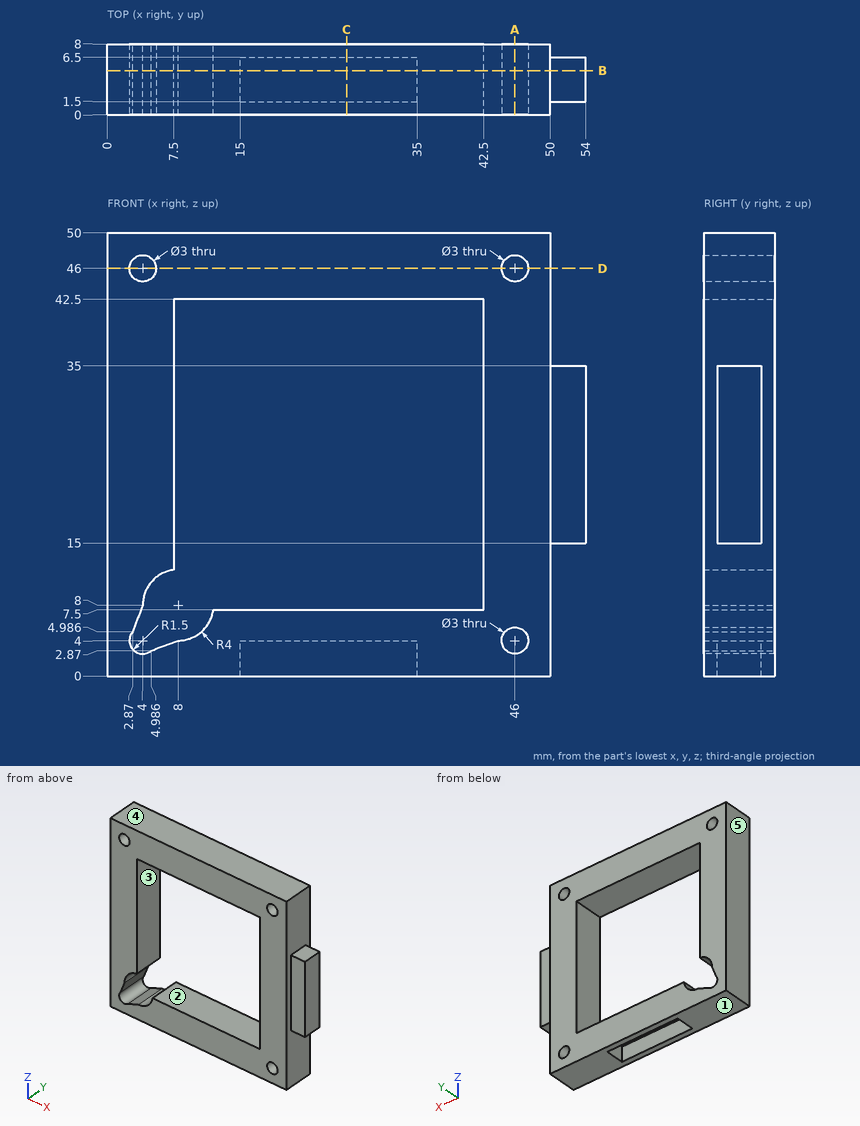
Print and shaded views of the part. All mm, measured from the part's lowest x, y and z. A direction names the side the tool comes from. Give positions to 0.01 mm unless a question says otherwise; leave off trailing zeros. Loops run counter-clockwise (first coordinate to the right, second up) from the corner with the lowest first, then second, coordinate; pieces in that order, holes last. Notation, with made-up numbers: (-37.5, 74) - (11.5, 74) arc R17 ccw to (11.5, 102) - close; hole circle Ø8 at (3.25, -20.5). An arc over 180 degrees is marked (long way). Use a Markdown table: item, result.
(1) Band-saw the part on C-C (x = 27). Give the cut face in (y, z), and give its area (3 significant figures).
Taken from the geometry:
| item | result |
|---|---|
| outline | (0, 0) - (1.5, 0) - (1.5, 4) - (6.5, 4) - (6.5, 0) - (8, 0) - (8, 7.5) - (0, 7.5) - close; (0, 42.5) - (8, 42.5) - (8, 50) - (0, 50) - close |
| area | 100 mm2 |
(2) Band-saw the part on B-B (y = 5). Give the cut face in (x, z), and give its area (3 significant figures).
Taken from the geometry:
| item | result |
|---|---|
| outline | (0, 0) - (15, 0) - (15, 4) - (35, 4) - (35, 0) - (50, 0) - (50, 15) - (54, 15) - (54, 35) - (50, 35) - (50, 50) - (0, 50) - close; hole circle Ø3 at (4, 46); hole (2.87, 4.99) arc R1.5 ccw to (4.99, 2.87) - (8, 4) arc R4 ccw to (11.97, 7.5) - (42.5, 7.5) - (42.5, 42.5) - (7.5, 42.5) - (7.5, 11.97) arc R4 ccw to (4, 8) - close; hole circle Ø3 at (46, 4); hole circle Ø3 at (46, 46) |
| area | 1,210 mm2 |
(3) Pull direction X, two halves, no side cores. Call the marked faces 3, 4 and 5: +X half, -X half, draft (parallel to the pull), parting line (faces both ways), or undercut.
Taken from the geometry:
| item | result |
|---|---|
| face 3 | undercut |
| face 4 | draft |
| face 5 | -X half |
(4) Band-saw the part on D-D (z = 46). Give the cut face in (x, y).
Taken from the geometry:
| item | result |
|---|---|
| outline | (0, 0) - (2.5, 0) - (2.5, 8) - (0, 8) - close; (5.5, 0) - (44.5, 0) - (44.5, 8) - (5.5, 8) - close; (47.5, 0) - (50, 0) - (50, 8) - (47.5, 8) - close |
(5) Drop flat-ended pins along their axis: pin 1 Ø1.2 at (x, z) = (52, 24) entering from +Y; pin 2 Ø4.5 at (x, y) = (52.5, 4) entering from -Z; pin 3 Ø2 at (y, z) = (5.5, 13.5) entering from +X. Give the stop position or say it passes through.
Taken from the geometry:
| item | result |
|---|---|
| pin 1 | y = 6.5 |
| pin 2 | z = 15 |
| pin 3 | x = 50 |
(6) Which spindle directions (+Z, -Z, +X, -X, +Y, -Y) get a long thin tool onto all of the face, cutting with end or side? Do the marked faces 1 and 2. Say none if no direction does.
Taken from the geometry:
| item | result |
|---|---|
| face 1 | -Z, +X, -X, +Y, -Y |
| face 2 | +Y, -Y |
(7) Band-saw the part on A-A (x = 46). Give the cut face in (y, z), and give its area (3 significant figures).
Taken from the geometry:
| item | result |
|---|---|
| outline | (0, 0) - (8, 0) - (8, 2.5) - (0, 2.5) - close; (0, 5.5) - (8, 5.5) - (8, 44.5) - (0, 44.5) - close; (0, 47.5) - (8, 47.5) - (8, 50) - (0, 50) - close |
| area | 352 mm2 |
(8) Wall check: line 1 along X through (y, z) = (1.5, 46); line 2 along X through (y, z) = (4.5, 34.5); line 3 along Z through (x, y) = (20, 6.75). Give the ranges that are in metal, low to high.
Taken from the geometry:
| item | result |
|---|---|
| line 1 | 0 to 2.5, 5.5 to 44.5, 47.5 to 50 |
| line 2 | 0 to 7.5, 42.5 to 54 |
| line 3 | 0 to 7.5, 42.5 to 50 |
